Build history of the part. All positions in model axes, mm. Face numbers are marked on the shaded views. A direction names the side the tool comes from. Give positions to 0.01 mm unless a question says otherwise; leave off trailing zeros. Write each loop counter-clockwise with the first axis right and the second up, starting at its lowest first coordinate (ties: lowest second). Pieces come first, ordered by that corner, then holes. Notation, with made-up numbers: (53.25, 1.5) -> (73.25, 1.5) arc R32 cw to (73.25, 32.5) -> close; hole circle Ø5 at (75.5, 78). An arc over 180 degrees is marked (long way). Put each result on its own line as item: value.
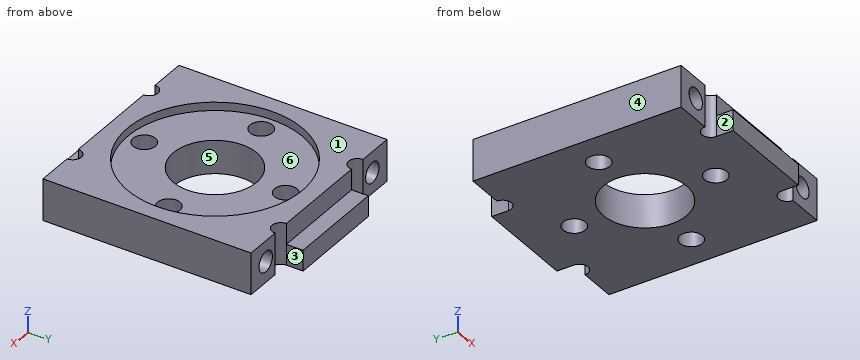
Autodesk Inventor part; units mm, degrees
ref_plane "YZ Plane" through (0, 0, 0) normal (1, 0, 0) x (0, 1, 0)
ref_plane "XZ Plane" through (0, 0, 0) normal (0, 1, 0) x (-1, 0, 0)
ref_plane "XY Plane" through (0, 0, 0) normal (0, 0, 1) x (1, 0, 0)
sketch "スケッチ1" plane through (0, 0, 0) normal (0, 0, 1) x (1, 0, 0)
  line L0 (12.5, -12.5) -> (12.5, 12.5) construction
  line L1 (-12.5, 12.5) -> (-12.5, -12.5) construction
  line L2 (-12.5, -12.5) -> (12.5, 12.5) construction
  line L3 (12.5, -12.5) -> (-12.5, 12.5) construction
  line L4 (-8.1, 12.5) -> (-12.5, 12.5)
  line L5 (-12.5, 12.5) -> (-12.5, 8.9019)
  line L6 (8.1, 12.5) -> (12.5, 12.5)
  line L7 (12.5, 12.5) -> (12.5, 8.1)
  line L8 (-12.5, -7.2981) -> (-12.5, -12.5)
  line L9 (-12.5, -12.5) -> (-8.1, -12.5)
  line L10 (8.1, -12.5) -> (12.5, -12.5)
  line L11 (12.5, -12.5) -> (12.5, -8.1)
  line L12 (-6, 12.5) -> (-6, 14.5)
  line L13 (-6, 14.5) -> (6, 14.5)
  line L14 (6, 14.5) -> (6, 12.5)
  arc A0 (-8.1, 12.5) -> (-6, 12.5) centre (-7.05, 12.5) ccw
  arc A1 (6, 12.5) -> (8.1, 12.5) centre (7.05, 12.5) ccw
  line L15 (0, 12.5) -> (0, 0) construction
  line L16 (0, 0) -> (12.5, 0) construction
  line L17 (-6, -12.5) -> (-6, -14.5)
  line L18 (-6, -14.5) -> (6, -14.5)
  line L19 (6, -14.5) -> (6, -12.5)
  arc A2 (-6, -12.5) -> (-8.1, -12.5) centre (-7.05, -12.5) ccw
  arc A3 (8.1, -12.5) -> (6, -12.5) centre (7.05, -12.5) ccw
  line L20 (-11.35, 12.5) -> (-8.25, 12.5) construction
  line L21 (-8.25, 12.5) -> (-8.25, 8.5) construction
  line L22 (-8.25, 8.5) -> (-11.35, 8.5) construction
  line L23 (-11.35, 8.5) -> (-11.35, 12.5) construction
  line L24 (-12.5, 6.7519) -> (-12.5, 9.8519) construction
  line L25 (-9.8, 12.5) -> (-9.8, 8.5) construction
  line L26 (-12.5, -12.5) -> (-12.5, 12.5)
  line L27 (12.5, -12.5) -> (12.5, 12.5)
  line L28 (0, -14.5) -> (0, 14.5) construction
  circle A4 centre (0, -8.5) radius 1.35
  circle A5 centre (8.5, 0) radius 1.35
  circle A6 centre (0, 8.5) radius 1.35
  circle A7 centre (-8.5, 0) radius 1.35
  circle A8 centre (0, 0) radius 5.01
  circle A9 centre (0, 0) radius 10.51
  line L29 (-6, 12.5) -> (6, 12.5)
  line L30 (-6, -12.5) -> (6, -12.5)
  dimension "d0" = 25
  dimension "d1" = 1.05
  dimension "d3" = 6.5
  dimension "d4" = 3.1
  dimension "d6" = 4
  dimension "d18" = 2.7
  dimension "d46" = 25
  dimension "d58" = 2.7
  dimension "d59" = 8.5
  dimension "d62" = 360
  dimension "d64" = 10.02
  dimension "d65" = 21.02
  dimension "d68" = 2
extrude "押し出し1" add sketch "スケッチ1" along normal blind 5 contours A0 L29 A1 L6 L7 L27 L11 L10 A3 L30 A2 L9 L8 L26 L5 L4
sketch "スケッチ2" plane through (-12.5, -12.5, 5) normal (0, -1, 0) x (1, 0, 0)
  line L0 (12.5, 0) -> (12.5, -5.2657) construction
  line L1 (0, -2.5) -> (22.3, -2.5) construction
  line L2 (25, -5) -> (25, 0)
  line L3 (0, -5) -> (0, 0)
  line L4 (0, 0) -> (4.4, 0)
  point P0 (12.5, -5)
  point P1 (2.7, -2.5)
  dimension "d56" = 2.7
  dimension "d57" = 2.7
  dimension "d69" = 2.5
hole "穴1" at (-9.8, -12.5, 2.5) at (9.8, -12.5, 2.5) direction (0, 1, 0) diameter 2.459 depth 8.8
pattern_circular "円形状パターン1" count 2 over 360 about axis through (0, 0, -10) along (0, 0, 1) of "穴1"
extrude "押し出し2" add sketch "スケッチ1" along normal blind 4 contours A9
extrude "押し出し3" add sketch "スケッチ1" along normal blind 2.5 contours L12 L13 L14 L29 | L30 L19 L18 L17
equation "\"d57\" = d56"
properties part number "Head_horn_frame" material "アセタール樹脂、黒"
1) Wall check: L1, parallel to Y at x = 0, z = 0.9; L2, parallel to Y at x = 0, z = 2.85; L3, parallel to Y at x = 8.5, z = 2.05. Give the ranges that are in metal, low to high.
Filled sheet:
L1: -14.5 to -9.85, -7.15 to -5.01, 5.01 to 7.15, 9.85 to 14.5
L2: -12.5 to -9.85, -7.15 to -5.01, 5.01 to 7.15, 9.85 to 12.5
L3: -12.5 to -1.35, 1.35 to 12.5
2) Slice it at C-C (x = 9.25). Write the cut outline in (y, z).
Filled sheet:
outline: (-12.5, 0) -> (-1.12, 0) -> (-1.12, 4) -> (-4.99, 4) -> (-4.99, 5) -> (-12.5, 5) -> (-12.5, 3.6) -> (-4.99, 3.6) -> (-4.99, 1.4) -> (-12.5, 1.4) -> close; (1.12, 0) -> (12.5, 0) -> (12.5, 1.4) -> (4.99, 1.4) -> (4.99, 3.6) -> (12.5, 3.6) -> (12.5, 5) -> (4.99, 5) -> (4.99, 4) -> (1.12, 4) -> close
3) Slice it at B-B (y = -4.5). Write the cut outline in (x, z).
Filled sheet:
outline: (-12.5, 0) -> (-2.2, 0) -> (-2.2, 4) -> (-9.5, 4) -> (-9.5, 5) -> (-12.5, 5) -> close; (2.2, 0) -> (12.5, 0) -> (12.5, 5) -> (9.5, 5) -> (9.5, 4) -> (2.2, 4) -> close; hole (-9.5, 1.31) -> (-9.5, 3.69) arc R1.23 ccw (long way) to start; hole (9.5, 1.31) arc R1.23 ccw (long way) to (9.5, 3.69) -> close
4) Tool access for the marked faces 1 and 2: list every direction of +Z, -Z, +X, -X, +Y, -Y with a clear straight run to the whole face (end or side of a thin tool).
Filled sheet:
face 1: +Z, +X, -X, +Y, -Y
face 2: +Z, -Z, -X, -Y
5) Slice it at D-D (y = 8.5). Write the cut outline in (x, z).
Filled sheet:
outline: (-12.5, 0) -> (-1.35, 0) -> (-1.35, 4) -> (-6.18, 4) -> (-6.18, 5) -> (-12.5, 5) -> close; (1.35, 0) -> (12.5, 0) -> (12.5, 5) -> (6.18, 5) -> (6.18, 4) -> (1.35, 4) -> close; hole circle Ø2.46 at (-9.8, 2.5); hole circle Ø2.46 at (9.8, 2.5)
6) Pin check, flat tips, straight feed: pin 1 (0.6 mm diameter, centred on y = 13.5, z = 1.5, fed in from +X); pin 2 (2 mm diameter, centred on x = 9.8, z = 2.5, fed in from -Y); pin 3 (1 mm diameter, centred on x = 10, z = 3, fed in from -Y). Stop position of each tip, or through.
Filled sheet:
pin 1: x = 6
pin 2: y = -5.75
pin 3: y = -4.5
7) Pull direction X, two halves, no side cores. Call the marked faces 3, 4, 5 and 6: released by +X, released by -X, zero draft, split by the parting line, or undercut.
Filled sheet:
face 3: released by +X
face 4: released by -X
face 5: undercut
face 6: undercut
8) Slice it at A-A (x = 0). Write the cut outline in (y, z), plus the area to 3 significant figures.
Filled sheet:
outline: (-14.5, 0) -> (-9.85, 0) -> (-9.85, 4) -> (-10.51, 4) -> (-10.51, 5) -> (-12.5, 5) -> (-12.5, 2.5) -> (-14.5, 2.5) -> close; (-7.15, 0) -> (-5.01, 0) -> (-5.01, 4) -> (-7.15, 4) -> close; (5.01, 0) -> (7.15, 0) -> (7.15, 4) -> (5.01, 4) -> close; (9.85, 0) -> (14.5, 0) -> (14.5, 2.5) -> (12.5, 2.5) -> (12.5, 5) -> (10.51, 5) -> (10.51, 4) -> (9.85, 4) -> close
area: 52.3 mm2
